```python
from build123d import *

# Parameters (mm, degrees)
F0_W     = 13
F0_H     = 28
F1_DEPTH = 2
F2_R     = 2
F3_R     = 2


with BuildPart() as f1:
    # F0 (on Front) → F1 (new body)
    with BuildSketch(Plane.XZ):
        Polygon((-8.465854, 10.590909), (-6.211373, 10.590909), (6.788627, 10.590909), (8.534146, 10.590909), (8.534146, 16.590909), (-8.465854, 16.590909), align=None)
        with Locations((0.288627, -3.409091)):
            Rectangle(F0_W, F0_H)
    extrude(amount=F1_DEPTH)

    # F2
    f2_edges = [f1.edges().sort_by_distance(p)[0] for p in [
        (-8.465854, -1, 16.590909),
        (-6.211373, -1, -17.409091),
    ]]
    fillet(f2_edges, radius=F2_R)

    # F3
    f3_edges = [f1.edges().sort_by_distance(p)[0] for p in [
        (8.534146, -1, 16.590909),
        (6.788627, -1, -17.409091),
    ]]
    fillet(f3_edges, radius=F3_R)


solid = f1.part
```
Input: part model. Units: mm. Frame: model coordinates. A direction names the side the tool comes from. Coordinates: 2 decimals unless noted, no trailing zeros. Write each loop counter-clockwise with the first axis right and the second up, starting at its lowest first coordinate (ties: lowest second). Pieces come first, ordered by that corner, then holes. Notation, with made-up numbers: (18, -36.5) -> (48, -36.5) arc R7 ccw to (48, -28.5) -> close; hole circle Ø7 at (-40, 39.5). An arc over 180 degrees is marked (long way). Write each question's results on one line, items separated by ' | '.
Item 1: Section query A-A on y = -1.15. Return loops of the section in (x, z).
Conclusion:
outline: (-8.47, 10.59) -> (-6.21, 10.59) -> (-6.21, -15.41) arc R2 ccw to (-4.21, -17.41) -> (4.79, -17.41) arc R2 ccw to (6.79, -15.41) -> (6.79, 10.59) -> (8.53, 10.59) -> (8.53, 14.59) arc R2 ccw to (6.53, 16.59) -> (-6.47, 16.59) arc R2 ccw to (-8.47, 14.59) -> close
Item 2: Section query C-C on x = -7.5. Return loops of the section in (y, z), plus the area to 3 significant figures.
Conclusion:
outline: (-2, 10.59) -> (0, 10.59) -> (0, 16.3) -> (-2, 16.3) -> close | area: 11.4 mm^2
Item 3: Pin query (flat end, axial travel): pin 1 Ø2 at (x, z) = (-2.5, -7) entering from +Y. Return the tip coordinate at first contact, or that it passes through.
Conclusion:
pin 1: stops at y = 0
Item 4: Set-up query: faces 1 (the flat face through (6.789, -1, -3)), 2 (the flat face through (-6.211, -1, -3)), 3 (the flat face through (0, -1, -17.409)). Return all of +Z, -Z, +X, -X, +Y, -Y with unobstructed straight access to the full face (end or side cutting, diameter ignored); none if empty.
Conclusion:
face 1: -Z, +X, +Y, -Y | face 2: -Z, -X, +Y, -Y | face 3: -Z, +X, -X, +Y, -Y
Item 5: Material intervals for probe 1 along Z at (x, y) = (-6.25, -1.05); probe 2 along X at (y, z) = (-0.15, 7); probe 3 along Z at (x, y) = (5.5, -1.85), sorted ascending.
Conclusion:
probe 1: z = 10.59 to 16.59 | probe 2: x = -6.21 to 6.79 | probe 3: z = -17.28 to 16.59
Item 6: Section query B-B on z = -11. Return loops of the section in (x, y), plus the area to 3 significant figures.
Conclusion:
outline: (-6.21, -2) -> (6.79, -2) -> (6.79, 0) -> (-6.21, 0) -> close | area: 26.0 mm^2
